```python
from build123d import *

# Parameters (mm, degrees)
SKETCH24_W               = 463
SKETCH24_H               = 506
BASE_FLANGE1_DEPTH       = 1.51892
SKETCH33_W               = 1.5
SKETCH33_H               = 4
SKETCH33_R               = 2.5
SKETCH33_R_2             = 1.5
SKETCH33_R_3             = 5
CUT_EXTRUDE1_DEPTH       = 1.51892
SKETCH35_R               = 1.513178902
SKETCH35_R_2             = 1.149873802
CUT_EXTRUDE3_DEPTH       = 10
M3_CLEARANCE_HOLE1_D     = 3.6
M3_CLEARANCE_HOLE1_DEPTH = 11.938
M3_CLEARANCE_HOLE1_TIP   = 1.081549114


# Sheet-metal steps are written as plain solids
with BuildPart() as part:
    # Sketch24 → Base-Flange1 (new body)
    with BuildSketch(Plane(origin=(0, 0, 0), x_dir=(1, 0, 0), z_dir=(0, 1, 0))):
        with Locations((0, -172.1425)):
            Rectangle(SKETCH24_W, SKETCH24_H)
    extrude(amount=-BASE_FLANGE1_DEPTH)

    # Sketch33 → Cut-Extrude1 (cut)
    with BuildSketch(Plane.XZ.offset(1.51892)):
        with BuildLine():
            Line((136.5, 375), (-136.5, 375))
            ThreePointArc((-136.5, 375), (-154.17766953, 367.67766953), (-161.5, 350))
            Line((-161.5, 350), (-161.5, 335))
            Line((-161.5, 335), (-169.5, 335))
            Line((-169.5, 335), (-169.5, 345))
            Line((-169.5, 345), (-173.5, 345))
            Line((-173.5, 345), (-173.5, 335))
            Line((-173.5, 335), (-181.5, 335))
            Line((-181.5, 335), (-181.5, 65))
            Line((-181.5, 65), (-173.5, 65))
            Line((-173.5, 65), (-173.5, 55))
            Line((-173.5, 55), (-169.5, 55))
            Line((-169.5, 55), (-169.5, 65))
            Line((-169.5, 65), (-161.5, 65))
            Line((-161.5, 65), (-161.5, 25))
            ThreePointArc((-161.5, 25), (-154.17766953, 7.32233047), (-136.5, 0))
            Line((-136.5, 0), (136.5, 0))
            ThreePointArc((136.5, 0), (154.17766953, 7.32233047), (161.5, 25))
            Line((161.5, 25), (161.5, 65))
            Line((161.5, 65), (169.5, 65))
            Line((169.5, 65), (169.5, 55))
            Line((169.5, 55), (173.5, 55))
            Line((173.5, 55), (173.5, 65))
            Line((173.5, 65), (181.5, 65))
            Line((181.5, 65), (181.5, 335))
            Line((181.5, 335), (173.5, 335))
            Line((173.5, 335), (173.5, 345))
            Line((173.5, 345), (169.5, 345))
            Line((169.5, 345), (169.5, 335))
            Line((169.5, 335), (161.5, 335))
            Line((161.5, 335), (161.5, 350))
            ThreePointArc((161.5, 350), (154.17766953, 367.67766953), (136.5, 375))
        make_face()
        with Locations((-176.25, 60)):
            Rectangle(SKETCH33_W, SKETCH33_H)
        with Locations((-166.75, 60)):
            Rectangle(SKETCH33_W, SKETCH33_H)
        with Locations((176.25, 60)):
            Rectangle(SKETCH33_W, SKETCH33_H)
        with Locations((166.75, 60)):
            Rectangle(SKETCH33_W, SKETCH33_H)
        with Locations((176.25, 340)):
            Rectangle(SKETCH33_W, SKETCH33_H)
        with Locations((166.75, 340)):
            Rectangle(SKETCH33_W, SKETCH33_H)
        with Locations((-166.75, 340)):
            Rectangle(SKETCH33_W, SKETCH33_H)
        with Locations((-176.25, 340)):
            Rectangle(SKETCH33_W, SKETCH33_H)
        with BuildLine():
            Line((195, -55.8575), (195, -80.8575))
            Line((195, -80.8575), (218, -80.8575))
            Line((218, -80.8575), (218, -55.8575))
            ThreePointArc((218, -55.8575), (206.5, -44.3575), (195, -55.8575))
        make_face()
        with BuildLine():
            ThreePointArc((-156.5, -55.8575), (-174.17766953, -63.17983047), (-181.5, -80.8575))
            Line((-181.5, -80.8575), (181.5, -80.8575))
            ThreePointArc((181.5, -80.8575), (174.17766953, -63.17983047), (156.5, -55.8575))
            Line((156.5, -55.8575), (-156.5, -55.8575))
        make_face()
        with BuildLine():
            Line((-218, -55.8575), (-218, -80.8575))
            Line((-218, -80.8575), (-195, -80.8575))
            Line((-195, -80.8575), (-195, -55.8575))
            ThreePointArc((-195, -55.8575), (-206.5, -44.3575), (-218, -55.8575))
        make_face()
        with Locations(Location((-206.5, 407.8575, 0), (0, 0, 270))):
            Circle(SKETCH33_R)
        with Locations(Location((-154, 391.8575, 0), (0, 0, 270))):
            Circle(SKETCH33_R)
        with Locations(Location((-138, 407.8575, 0), (0, 0, 270))):
            Circle(SKETCH33_R)
        with Locations(Location((138, 407.8575, 0), (0, 0, 270))):
            Circle(SKETCH33_R)
        with Locations(Location((154, 391.8575, 0), (0, 0, 270))):
            Circle(SKETCH33_R)
        with Locations(Location((206.5, 407.8575, 0), (0, 0, 270))):
            Circle(SKETCH33_R)
        with Locations(Location((154, -30.715, 0), (0, 0, 270))):
            Circle(SKETCH33_R)
        with Locations(Location((122, -30.715, 0), (0, 0, 270))):
            Circle(SKETCH33_R)
        with Locations(Location((191, -40.3575, 0), (0, 0, 270))):
            Circle(SKETCH33_R_2)
        with Locations(Location((191, -71.3575, 0), (0, 0, 270))):
            Circle(SKETCH33_R_2)
        with Locations(Location((222, -40.3575, 0), (0, 0, 270))):
            Circle(SKETCH33_R_2)
        with Locations(Location((222, -71.3575, 0), (0, 0, 270))):
            Circle(SKETCH33_R_2)
        with Locations(Location((-154, -30.715, 0), (0, 0, 270))):
            Circle(SKETCH33_R)
        with Locations(Location((-122, -30.715, 0), (0, 0, 270))):
            Circle(SKETCH33_R)
        with Locations(Location((-222, -40.3575, 0), (0, 0, 270))):
            Circle(SKETCH33_R_2)
        with Locations(Location((-222, -71.3575, 0), (0, 0, 270))):
            Circle(SKETCH33_R_2)
        with Locations(Location((-191, -71.3575, 0), (0, 0, 270))):
            Circle(SKETCH33_R_2)
        with Locations(Location((-191, -40.3575, 0), (0, 0, 270))):
            Circle(SKETCH33_R_2)
        with Locations(Location((0, -10.8575, 0), (0, 0, 270))):
            Circle(SKETCH33_R_3)
    extrude(amount=-CUT_EXTRUDE1_DEPTH, mode=Mode.SUBTRACT)

    # Sketch35 → Cut-Extrude3 (cut)
    with BuildSketch(Plane.XZ.offset(1.51892)):
        with Locations(Location((-206.607994526, -30.137642513, 0), (0, 0, 270))):
            Circle(SKETCH35_R)
        with Locations(Location((205.958496696, -31.650821415, 0), (0, 0, 270))):
            Circle(SKETCH35_R_2)
    extrude(amount=-CUT_EXTRUDE3_DEPTH, mode=Mode.SUBTRACT)

    # M3 Clearance Hole1
    with Locations(Plane(origin=(0, -1.51892, 0), x_dir=(-1, 0, 0), z_dir=(0, -1, 0))):
        with Locations((217.84, -417.1425), (-217.8375, -417.1425), (217.84, -345.341666667), (217.84, -273.540833333), (217.84, -201.74), (217.84, -129.939166667), (217.84, -58.138333333), (-217.8375, -58.138333333), (-217.8375, -129.939166667), (-217.8375, -201.74), (-217.8375, -273.540833333), (-217.8375, -345.341666667), (145.227083333, 13.6625), (72.614166667, 13.6625), (0.00125, 13.6625), (-72.611666667, 13.6625), (-145.224583333, 13.6625), (217.84, 13.6625), (-217.8375, 13.6625)):
            Hole(M3_CLEARANCE_HOLE1_D / 2, depth=M3_CLEARANCE_HOLE1_DEPTH)
            with Locations((0, 0, -(M3_CLEARANCE_HOLE1_DEPTH + M3_CLEARANCE_HOLE1_TIP / 2))):  # 118° drill point
                Cone(0, M3_CLEARANCE_HOLE1_D / 2, M3_CLEARANCE_HOLE1_TIP, mode=Mode.SUBTRACT)


solid = part.part
```
Geometry check sheet. Reference: the model listing, model coordinates, mm. A direction names the side the tool comes from. Round coordinates to 2 decimals unless told otherwise and drop trailing zeros. Order: outer loops, then holes, each group sorted by start corner. A loop starts at its lowest first (then second) coordinate and runs counter-clockwise, first axis right, second up. Notation, with made-up numbers: M 6,72.25 L 56,72.25 A34 ccw 56,108.25 Z; hole C 38,1 d8. An arc over 180 degrees is marked long. Answer as CSV lines item,"result".
1) Gauge pin test, flat ends, axial feed: pin 1 Ø3 at (x, z) = (217.84, 273.54) entering from +Y; pin 2 Ø0.5 at (x, y) = (-172, -0.5) entering from -Z; pin 3 Ø5 at (x, z) = (-191, -40.36) entering from -Y; pin 4 Ø0.8 at (x, y) = (-167, -1) entering from -Z. Record the tip position at first contact, or that the pin passes through.
Entries:
pin 1,"through"
pin 2,"z = -61.44"
pin 3,"y = -1.52"
pin 4,"z = -58.36"
2) Sectioned sample at C-C on y = -0.7. Give the number of separate pieces and of enclosed holes in the cut face, and give its area (3 significant figures).
Entries:
separate pieces,"1"
enclosed holes,"48"
area,"91,800 mm2"
3) Mould release check, pull along Z, two halves, no side actions. Record for faces 4 (the face through (-3, 0, 393)), 5 (the face through (154.371, -0.77, 367.482)), 6 (the face through (174.371, -0.77, -63.375)): +Z half, -Z half, draft (parallel to the pull), parting line (faces both ways), or undercut.
Entries:
face 4,"draft"
face 5,"undercut"
face 6,"-Z half"
4) Sectioned sample at A-A on z = 155.5. Record the cut outline in (x, y).
Entries:
outline,"M -231.5,-1.52 L -181.5,-1.52 L -181.5,0 L -231.5,0 Z; M 181.5,-1.52 L 231.5,-1.52 L 231.5,0 L 181.5,0 Z"
5) Thickness scan on probe 1 along X at (y, z) = (-0.1, -55); probe 2 along Z at (x, y) = (222, -0.7); probe 3 along X at (y, z) = (-0.35, 317.5). Record the ranges inside material, lowest first. Write a range as [from, to].
Entries:
probe 1,"[-231.5, -217.97], [-195.03, 195.03], [217.97, 231.5]"
probe 2,"[-80.86, -72.86], [-69.86, -41.86], [-38.86, 425.14]"
probe 3,"[-231.5, -181.5], [181.5, 231.5]"
6) Tool access check on faces 1 (the face through (-154.371, -0.77, 7.518)), 2 (the face through (-3, -1.519, 393)), 3 (the face through (-173.982, -0.77, -62.987)). Record the directions out of +Z, -Z, +X, -X, +Y, -Y that give a thin tool (end or side, any length) a straight path to the whole face; none if there is none.
Entries:
face 1,"+Y, -Y"
face 2,"+Z, -Z, +X, -X, -Y"
face 3,"-Z, +Y, -Y"
7) Sectioned sample at B-B on x = 26.5. Record the cut outline in (y, z), and give its area (3 significant figures).
Entries:
outline,"M -1.52,-55.86 L 0,-55.86 L 0,0 L -1.52,0 Z; M -1.52,375 L 0,375 L 0,425.14 L -1.52,425.14 Z"
area,"161 mm2"
